The model under review builds one solid part; all positions refer to its coordinate system, in mm. A direction names the side the tool comes from. Give positions to 0.01 mm unless a question says otherwise; leave off trailing zeros. Order: outer loops, then holes, each group sorted by start corner. A loop starts at its lowest first (then second) coordinate and runs counter-clockwise, first axis right, second up. Notation, with made-up numbers: (45, -26) - (60, -26) arc R7 ccw to (60, -20) - close; hole circle Ø10 at (33.25, 19). An arc over 180 degrees is marked (long way). Use a Markdown table: item, result. Add a question column.
```python
from build123d import *

# Parameters (mm, degrees)
SKETCH1_R           = 5
SKETCH1_R_2         = 2.630242902
BOSS_EXTRUDE1_DEPTH = 5


with BuildPart() as part:
    # Sketch1 → Boss-Extrude1 (new body)
    with BuildSketch(Plane.XY):
        with BuildLine():
            ThreePointArc((-132.270242639, 188.16105578), (-148.132436646, 175.945392703), (-162.872207874, 162.396563703))
            Line((-162.872207874, 162.396563703), (-153.220049521, 152.772593049))
            ThreePointArc((-153.220049521, 152.772593049), (-144.175949012, 161.335502877), (-134.654137313, 169.363845217))
            ThreePointArc((-134.654137313, 169.363845217), (-91.974174204, 129.962156064), (-76.195, 74.059651464))
            ThreePointArc((-76.195, 74.059651464), (-73.571522122, 67.708276367), (-67.230563194, 65.059721728))
            ThreePointArc((-67.230563194, 65.059721728), (-23.540861603, 45.781560748), (-7.974687844, 0.635888194))
            ThreePointArc((-7.974687844, 0.635888194), (-0.758972679, -7.963916152), (7.951244839, -0.881876127))
            ThreePointArc((7.951244839, -0.881876127), (-2.808500316, 37.921764044), (-31.962523765, 65.698328321))
            ThreePointArc((-31.962523765, 65.698328321), (-50.993465666, 81.748695293), (-61.871355452, 104.142054652))
            ThreePointArc((-61.871355452, 104.142054652), (-87.362753882, 154.285853019), (-132.270242639, 188.16105578))
        make_face()
        with Locations((-67.195, 74.059651464)):
            Circle(SKETCH1_R, mode=Mode.SUBTRACT)
        Circle(SKETCH1_R_2, mode=Mode.SUBTRACT)
    extrude(amount=BOSS_EXTRUDE1_DEPTH)


solid = part.part
```
Q1. We need section B-B (z = 3.95). Write out the cut boundary in (x, y) (3 decimals).
Q2. Wall thickness on probe 1 along Y at (x, z) = (-69.5, 0.75); probe 2 along X at (y, z) = (72.5, 3.55); probe 3 along X at (y, z) = (161.5, 0.75): over which ranges is each line inside the solid? List them lowest first.
Q3. We need section C-C (y = 129). Write out the cut boundary in (x, z).
Q4. Draft analysis for pull direction Y (two halves, no side actions). For faces 3 (the cylindrical face through (-0.34, 2.61, 2.46)), 4 (the flat face through (-72, 105, 5)), 5 (the cylindrical face through (-62.58, 72.14, 2.46)), 6 (the cylindrical face through (-86.855, 153.675, 2.465)), state which applies: pulls with the +Y half, pulls with the -Y half, needs draft (parallel to the pull), parting line crosses it, or undercut.
Q5. Clearance check with flat-ended pins moving along their axes: P1, Ø1, axis at y = 46.5, z = 3.5, coming from the -X side; P2, Ø1, axis at y = 59, z = 4.5, coming from the -X side; P3, Ø2, axis at x = -69.5, z = 4, coming from the -Y side. State where each tip first meets the part, or that it passes through.
Q6. Machinability: for faces 1 (the flat face through (-158.11, 157.65, 2.46)), 2 (the cylindrical face through (-144.306, 161.219, 2.465)), which of the approach directions +Z, -Z, +X, -X, +Y, -Y give a long, thin tool a straight path to every point of the face, cutting with its end or side? Answer none if there is none.
Q7. We need section D-D (x = -145). Write out the cut boundary in (y, z), plus the area to 3 significant figures.
Q8. We need section A-A (x = 0). Write out the cut boundary in (y, z).
Here are the results:
| question | item | result |
|---|---|---|
| 1 | outline | (-162.872, 162.397) - (-153.22, 152.773) arc R216.37 cw to (-134.654, 169.364) arc R106.915 cw to (-76.195, 74.06) arc R9 ccw to (-67.231, 65.06) arc R59.681 cw to (-7.975, 0.636) arc R8 ccw to (7.951, -0.882) arc R75.607 ccw to (-31.963, 65.698) arc R60 cw to (-61.871, 104.142) arc R124.915 ccw to (-132.27, 188.161) arc R230 ccw to start; hole circle Ø10 at (-67.195, 74.06); hole circle Ø5.26 at (0, 0) |
| 2 | probe 1 | 65.36 to 69.62, 78.5 to 125.99 |
| 2 | probe 2 | -76.06 to -71.95, -62.44 to -42.05 |
| 2 | probe 3 | -161.97 to -143.99, -121.59 to -93.9 |
| 3 | outline | (-91.39, 0) - (-70.93, 0) - (-70.93, 5) - (-91.39, 5) - close |
| 4 | face 3 | undercut |
| 4 | face 4 | needs draft |
| 4 | face 5 | undercut |
| 4 | face 6 | pulls with the +Y half |
| 5 | P1 | x = -24.69 |
| 5 | P2 | x = -42.31 |
| 5 | P3 | y = 65.15 |
| 6 | face 1 | +Z, -Z, -X, -Y |
| 6 | face 2 | +Z, -Z, -Y |
| 7 | outline | (160.6, 0) - (178.54, 0) - (178.54, 5) - (160.6, 5) - close |
| 7 | area | 89.7 mm2 |
| 8 | outline | (-8, 0) - (-2.63, 0) - (-2.63, 5) - (-8, 5) - close; (2.63, 0) - (32.8, 0) - (32.8, 5) - (2.63, 5) - close |
